The figure shows three views and two pictorial views of one solid part (mm, origin at its lowest corner). Answer the questions. Round coordinates to 2 decimals unless told otherwise and drop trailing zeros. Write each loop counter-clockwise with the first axis right and the second up, starting at its lowest first coordinate (ties: lowest second). Pieces come first, ordered by that corner, then holes. Notation, with made-up numbers: M 74.5,57.5 L 115.5,57.5 A13 ccw 115.5,65.5 Z; hole C 87.25,1 d4. An arc over 180 degrees is marked long. Use one line per item in the form item = value. Start each with the question number.
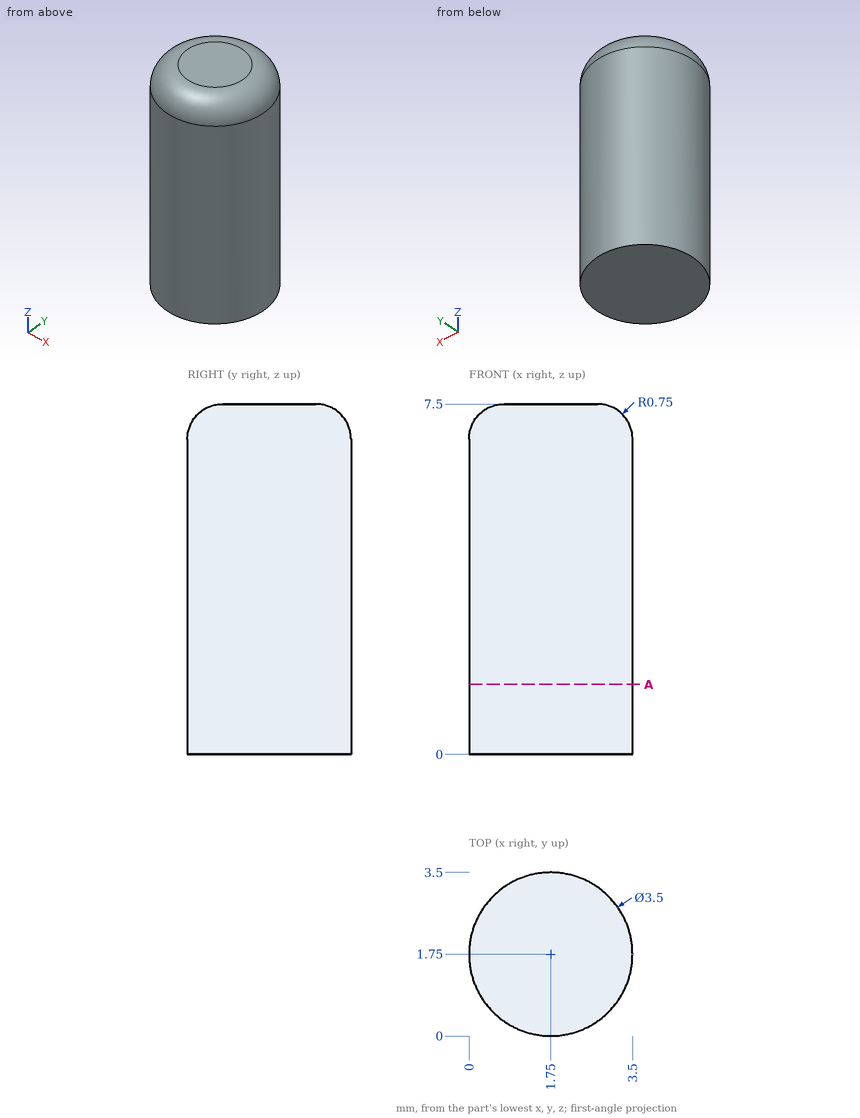
Q1. Straight lines are drawn through the part: line 1 (X direction, y = 2.8, z = 2); line 2 (Z direction, x = 1.4, y = 0.6); line 3 (Y direction, x = 0.3, z = 3.25). For each, find the intervals that lie inside material, in ascending order. Write a range as [from, to].
Q2. Find section A-A on z = 1.5. Write down the section's boundary in (x, y), and give its area (3 significant figures).
Q3. This flat-tipped pin is pushed along its axis until it touches: pin 1 Ø1.5 at (x, z) = (3, 6.5) entering from -Y. Where does it stop, or does it pass through?
Response:
q1.line_1 = [0.35, 3.15]
q1.line_2 = [0, 7.47]
q1.line_3 = [0.77, 2.73]
q2.outline = C 1.75,1.75 d3.5
q2.area = 9.62 mm²
q3.pin_1 = 0.07
